Can you work these out from the model? Positions are in its coordinate system, mm. Face numbers are marked on the shaded views. A direction names the side the tool comes from. Coordinates: 2 decimals unless noted, no trailing zeros. Order: outer loops, then holes, each group sorted by start corner. A loop starts at its lowest first (then second) coordinate and runs counter-clockwise, first axis right, second up. Notation, with made-up numbers: (39, 3.25) -> (75, 3.25) arc R19 ccw to (75, 30.25) -> close; hole circle Ø4 at (20, 70.25). An arc over 180 degrees is marked (long way). Write item = value, one per line.
```python
from build123d import *

# Parameters (mm, degrees)
SKETCH1_W           = 1058.297604825
SKETCH1_H           = 1375
BOSS_EXTRUDE4_DEPTH = 1000
SKETCH1_7_W         = 1058.297604825
SKETCH1_7_H         = 875
BOSS_EXTRUDE5_DEPTH = 875
SKETCH5_R           = 250
CUT_EXTRUDE1_DEPTH  = 1188
SKETCH6_R           = 187.5
CUT_EXTRUDE7_DEPTH  = 875
SKETCH7_R           = 237.5
CUT_EXTRUDE8_DEPTH  = 125
FILLET2_R           = 400


with BuildPart() as part:
    # Sketch1 → Boss-Extrude4 (new body)
    with BuildSketch(Plane(origin=(0, 0, 0), x_dir=(1, 0, 0), z_dir=(0, 1, 0))):
        with Locations((418.500975611, 243.415773734)):
            Rectangle(SKETCH1_W, SKETCH1_H)
    extrude(amount=BOSS_EXTRUDE4_DEPTH)

    # Sketch1_7 → Boss-Extrude5 (add)
    with BuildSketch(Plane(origin=(0, 0, 0), x_dir=(1, 0, 0), z_dir=(0, 1, 0))):
        with Locations((418.500975611, -881.584226266)):
            Rectangle(SKETCH1_7_W, SKETCH1_7_H)
    extrude(amount=BOSS_EXTRUDE5_DEPTH)

    # Sketch5 → Cut-Extrude1 (cut)
    with BuildSketch(Plane.XY.offset(1319.084226266)):
        with Locations((418.500975611, 437.5)):
            Circle(SKETCH5_R)
    extrude(amount=-CUT_EXTRUDE1_DEPTH, mode=Mode.SUBTRACT)

    # Sketch6 → Cut-Extrude7 (cut)
    with BuildSketch(Plane(origin=(0, 1000, 0), x_dir=(1, 0, 0), z_dir=(0, 1, 0))):
        with Locations(Location((418.500975611, 243.415773734, 0), (0, 0, 270))):
            Circle(SKETCH6_R)
    extrude(amount=-CUT_EXTRUDE7_DEPTH, mode=Mode.SUBTRACT)

    # Sketch7 → Cut-Extrude8 (cut)
    with BuildSketch(Plane(origin=(0, 0, 0), x_dir=(-1, 0, 0), z_dir=(0, -1, 0))):
        with Locations(Location((-418.500975611, 243.415773734, 0), (0, 0, 90))):
            Circle(SKETCH7_R)
    extrude(amount=-CUT_EXTRUDE8_DEPTH, mode=Mode.SUBTRACT)

    # Fillet2
    fillet2_edges = [part.edges().sort_by_distance(p)[0] for p in [
        (-110.647826802, 500, -930.915773734),
        (947.649778023, 500, -930.915773734),
    ]]
    fillet(fillet2_edges, radius=FILLET2_R)


solid = part.part
```
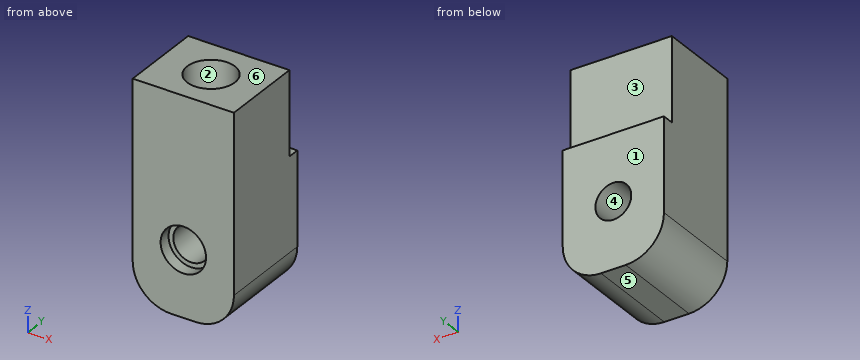
Item 1: I want a section at B-B, the plane y = 556.5. Please give me the cut outline in (x, z), plus the area to 3 significant figures.
A:
outline = (-110.65, -530.92) arc R400 ccw to (289.35, -930.92) -> (547.65, -930.92) arc R400 ccw to (947.65, -530.92) -> (947.65, 1319.08) -> (638.36, 1319.08) -> (638.36, 131.08) -> (198.64, 131.08) -> (198.64, 1319.08) -> (-110.65, 1319.08) -> close; hole circle Ø375 at (418.5, -243.42)
area = 1,680,000 mm2
Item 2: I want a section at A-A, the plane z = -409. Please give me the cut outline in (x, y).
A:
outline = (-110.65, 0) -> (248.24, 0) -> (248.24, 125) -> (330.53, 125) -> (330.53, 1000) -> (-110.65, 1000) -> close; (506.47, 125) -> (588.76, 125) -> (588.76, 0) -> (947.65, 0) -> (947.65, 1000) -> (506.47, 1000) -> close
Item 3: I want a section at C-C, the plane z = 742. Please give me the cut outline in (x, y), plus the area to 3 significant figures.
A:
outline = (-110.65, 0) -> (947.65, 0) -> (947.65, 875) -> (-110.65, 875) -> close; hole circle Ø500 at (418.5, 437.5)
area = 730,000 mm2
Item 4: If we mould it in two halves opening along Z, with no side actions, what happens to the marked faces 4, 5 and 6? For each: pulls with the +Z half, pulls with the -Z half, needs draft (parallel to the pull), parting line crosses it, or undercut.
A:
face_4 = undercut
face_5 = pulls with the -Z half
face_6 = pulls with the +Z half
Item 5: I'm going to push flat-ended pins straight in: P1, Ø4, axis at x = 420, z = 918.5, coming from the +Y side; P2, Ø1.5, axis at x = 658.5, y = 567, coming from the -Z side. Where does each tip first touch, or does it pass through?
A:
P1 = 875
P2 = -915.46
Item 6: I want a section at D-D, the plane x = 45. Please give me the cut outline in (y, z), plus the area to 3 significant figures.
A:
outline = (0, -847.6) -> (1000, -847.6) -> (1000, 444.08) -> (875, 444.08) -> (875, 1319.08) -> (0, 1319.08) -> close
area = 2,060,000 mm2
Item 7: For the marked faces 1, 2 and 3, which set-ups out of +Z, -Z, +X, -X, +Y, -Y let a thin tool reach every point of the face, with its end or its side?
A:
face_1 = +Z, -Z, +X, -X, +Y
face_2 = +Z
face_3 = +Z, +X, -X, +Y
Item 8: If I drill on probe 1 along X at (y, z) = (437, 596); probe 2 along Z at (x, y) = (426, 882.5); probe 3 along Y at (x, z) = (410.5, 941), over which ranges is the centre line in solid material (lowest first)?
A:
probe_1 = -110.65 to 168.5, 668.5 to 947.65
probe_2 = -930.92 to -430.77, -56.07 to 444.08
probe_3 = 0 to 187.63, 687.37 to 875
